Build history of the part. All positions in model axes, mm. Face numbers are marked on the shaded views. Round coordinates to 2 decimals unless told otherwise and drop trailing zeros. Order: outer loops, then holes, each group sorted by start corner. A loop starts at its lowest first (then second) coordinate and runs counter-clockwise, first axis right, second up. Notation, with made-up numbers: (-0.75, -21.75) -> (35.25, -21.75) arc R29 ccw to (35.25, 7.25) -> close; hole circle Ø5 at (15.5, 60.5). An arc over 180 degrees is marked (long way). Use a Markdown table: item, result. Add a question column.
Item 1: Probe L1, parallel to Y at x = 0, z = 9.5; L2, parallel to Y at x = 4.5, z = 5.25. List the from-to ranges inside material, lowest first.
Item 2: Slice it at C-C, the plane y = 0. Give the cut face in (x, z), plus the area to 4 significant figures.
Item 3: Slice it at B-B, the plane z = 7. Give the cut face in (x, y).
Item 4: Slice it at A-A, the plane x = 0. Give the cut face in (y, z).
Item 5: Two-plate mould, pull along X, no slides. Class the marked faces 1, 2 and 3: released by +X, released by -X, zero draft, split by the parting line, or undercut.
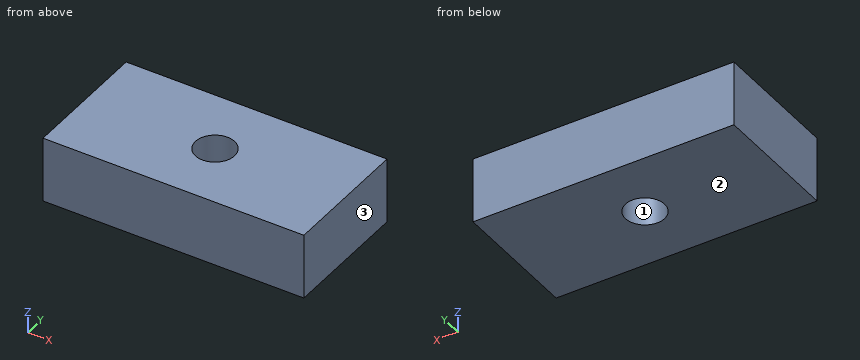
from build123d import *

# Parameters (mm, degrees)
SKICA1_W                 = 100
SKICA1_H                 = 50
P_IDAT_VYSUNUT_M1_DEPTH  = 25
ODEBRAT_VYSUNUT_M1_REACH = 27
SKICA2_R                 = 7.5


with BuildPart() as part:
    # Skica1 → Přidat vysunutím1 (new body)
    with BuildSketch(Plane.XY):
        Rectangle(SKICA1_W, SKICA1_H)
    extrude(amount=P_IDAT_VYSUNUT_M1_DEPTH)

    # Skica2 → Odebrat vysunutím1 (cut, up to next)
    with BuildSketch(Plane.XY.offset(25), mode=Mode.PRIVATE) as odebrat_vysunut_m1_sk1:
        Circle(SKICA2_R)
    odebrat_vysunut_m1_tool1 = extrude(odebrat_vysunut_m1_sk1.sketch, amount=-ODEBRAT_VYSUNUT_M1_REACH, mode=Mode.PRIVATE) & part.part
    add(odebrat_vysunut_m1_tool1.solids().sort_by_distance((0, 0, 25))[0], mode=Mode.SUBTRACT)


solid = part.part
Check sheet entries:
| question | item | result |
|---|---|---|
| 1 | L1 | -25 to -7.5, 7.5 to 25 |
| 1 | L2 | -25 to -6, 6 to 25 |
| 2 | outline | (-50, 0) -> (-7.5, 0) -> (-7.5, 25) -> (-50, 25) -> close; (7.5, 0) -> (50, 0) -> (50, 25) -> (7.5, 25) -> close |
| 2 | area | 2,125 mm2 |
| 3 | outline | (-50, -25) -> (50, -25) -> (50, 25) -> (-50, 25) -> close; hole circle Ø15 at (0, 0) |
| 4 | outline | (-25, 0) -> (-7.5, 0) -> (-7.5, 25) -> (-25, 25) -> close; (7.5, 0) -> (25, 0) -> (25, 25) -> (7.5, 25) -> close |
| 5 | face 1 | undercut |
| 5 | face 2 | zero draft |
| 5 | face 3 | released by +X |
